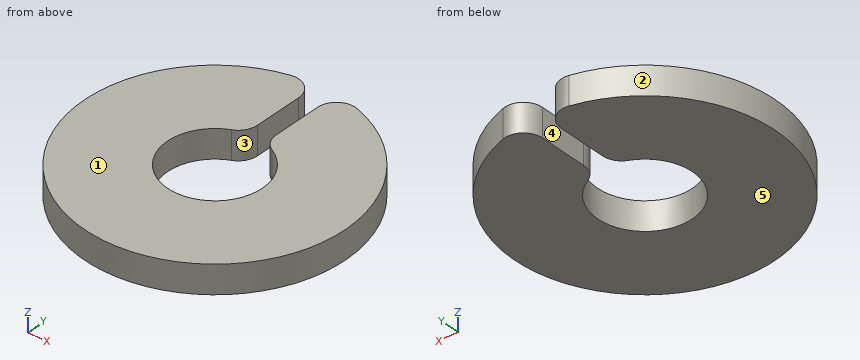
Autodesk Inventor part; units mm, degrees
ref_plane "YZ Plane" through (0, 0, 0) normal (1, 0, 0) x (0, 1, 0)
ref_plane "XZ Plane" through (0, 0, 0) normal (0, 1, 0) x (-1, 0, 0)
ref_plane "XY Plane" through (0, 0, 0) normal (0, 0, 1) x (1, 0, 0)
sketch "Sketch1" plane through (0, 0, 0) normal (0, 0, 1) x (1, 0, 0)
  arc A0 (-3.5106, 13.2943) -> (3.5106, 13.2943) centre (0, 0) ccw
  circle A1 centre (0, 0) radius 4.5 construction
  line L0 (-1, 11.3606) -> (-1, 3.5)
  line L1 (1, 3.5) -> (1, 11.3606)
  arc A2 (-1, 3.5) -> (1, 3.5) centre (0, 3.5) ccw
  line L2 (-9.75, -9.75) -> (9.75, -9.75) construction
  line L3 (9.75, -9.75) -> (9.75, 9.75) construction
  line L4 (9.75, 9.75) -> (-9.75, 9.75) construction
  line L5 (-9.75, 9.75) -> (-9.75, -9.75) construction
  line L6 (-9.75, -9.75) -> (9.75, 9.75) construction
  line L7 (9.75, -9.75) -> (-9.75, 9.75) construction
  arc A3 (-1, 11.3606) -> (-3.5106, 13.2943) centre (-3, 11.3606) ccw
  arc A4 (3.5106, 13.2943) -> (1, 11.3606) centre (3, 11.3606) ccw
  point P0 (0, 6.1182)
  point P1 (0, 4.5)
  point P2 (0, 2.5)
  point P3 (0, 2.5)
  dimension "d1" = 9
  dimension "d0" = 27.5
  dimension "d2" = 2
  dimension "d3" = 2
  dimension "d5" = 19.5
  dimension "d9" = 19.5
  dimension "d10" = 2
extrude "Extrusion1" add sketch "Sketch1" along normal blind 3
sketch "Sketch2" plane through (0, 0, 3) normal (0, 0, 1) x (1, 0, 0)
  circle A0 centre (0, 0) radius 5
  dimension "d11" = 10
extrude "Extrusion2" cut sketch "Sketch2" against normal through all
fillet "Fillet1" radius 2 2 edges at (-1, 4.899, 1.5) (1, 4.899, 1.5)
properties part number "FrontTerm"
Can you work these out from the model? Positions are in its coordinate system, mm. Face numbers are marked on the shaded views. A direction names the side the tool comes from. Round coordinates to 2 decimals unless told otherwise and drop trailing zeros. Loops run counter-clockwise (first coordinate to the right, second up) from the corner with the lowest first, then second, coordinate; pieces in that order, holes last. Notation, with made-up numbers: (84, 42.5) - (139, 42.5) arc R14 cw to (139, 66.5) - close; hole circle Ø8 at (58, 62). An arc over 180 degrees is marked (long way). Write item = value, one per line. Start each with the question number.
(1) If I drill on probe 1 along X at (y, z) = (0, 0.7); probe 2 along Y at (x, z) = (0, 1.4); probe 3 along X at (y, z) = (-4.5, 1.75), over which ranges is the centre line in solid material (lowest first)? Write a range as [from, to].
(2) For P1, Ø1.5, axis at y = 5, z = 1.5, coming from the +X side, with a flat end and sliding along its axis, tell me the tip position at first contact or that it passes through.
(3) If we section it at A-A (y = 0): Please give me the cut outline in (x, z), and give its area (3 significant figures).
(4) If we section it at B-B (z = 1.55): Please give me the cut outline in (x, y), and give its area (3 significant figures).
(5) For the marked faces 4 and 5, which set-ups out of +Z, -Z, +X, -X, +Y, -Y let a thin tool reach every point of the face, with its end or its side?
(6) If we section it at C-C (x = 0): Please give me the cut outline in (y, z), and give its area (4 significant figures).
(7) If we mould it in two halves opening along X, with no side actions, what happens to the marked faces 1, 2 and 3? For each: released by +X, released by -X, zero draft, split by the parting line, or undercut.
(8) If we section it at D-D (x = 6.5): Please give me the cut outline in (y, z).
Ans:
q1.probe_1 = [-13.75, -5], [5, 13.75]
q1.probe_2 = [-13.75, -5]
q1.probe_3 = [-12.99, -2.18], [2.18, 12.99]
q2.P1 = 13.08
q3.outline = (-13.75, 0) - (-5, 0) - (-5, 3) - (-13.75, 3) - close; (5, 0) - (13.75, 0) - (13.75, 3) - (5, 3) - close
q3.area = 52.5 mm²
q4.outline = (-3.51, 13.29) arc R13.75 ccw (long way) to (3.51, 13.29) arc R2 ccw to (1, 11.36) - (1, 6.32) arc R2 ccw to (2.14, 4.52) arc R5 cw (long way) to (-2.14, 4.52) arc R2 ccw to (-1, 6.32) - (-1, 11.36) arc R2 ccw to start
q4.area = 495 mm²
q5.face_4 = +Z, -Z, +Y
q5.face_5 = -Z, +X, -X, +Y, -Y
q6.outline = (-13.75, 0) - (-5, 0) - (-5, 3) - (-13.75, 3) - close
q6.area = 26.25 mm²
q7.face_1 = zero draft
q7.face_2 = split by the parting line
q7.face_3 = undercut
q8.outline = (-12.12, 0) - (12.12, 0) - (12.12, 3) - (-12.12, 3) - close
